```python
from build123d import *

# Parameters (mm, degrees)
F0_R     = 20
F1_DEPTH = 5
F2_W     = 5
F2_H     = 7.376282
F2_H_2   = 5
F3_DEPTH = 2


with BuildPart() as f1:
    # F0 (on Right) → F1 (new body)
    with BuildSketch(Plane.YZ):
        with BuildLine():
            Line((3.688141, 0), (3.688141, 32.210336))
            ThreePointArc((3.688141, 32.210336), (0, 75.898988), (-3.688141, 32.210336))
            Line((-3.688141, 32.210336), (-3.688141, 0))
            Line((-3.688141, 0), (3.688141, 0))
        make_face()
        with Locations((0, 53.898988)):
            Circle(F0_R, mode=Mode.SUBTRACT)
    extrude(amount=F1_DEPTH)

    # F2 (on Top) → F3 (join)
    with BuildSketch(Plane.XY):
        with Locations((2.5, 0)):
            Rectangle(F2_W, F2_H)
        with Locations((2.5, -6.188141)):
            Rectangle(F2_W, F2_H_2)
        with Locations((2.5, 6.188141)):
            Rectangle(F2_W, F2_H_2)
    extrude(amount=F3_DEPTH)


solid = f1.part
```
The model under review builds one solid part; all positions refer to its coordinate system, in mm. A direction names the side the tool comes from. Round coordinates to 2 decimals unless told otherwise and drop trailing zeros. Order: outer loops, then holes, each group sorted by start corner. A loop starts at its lowest first (then second) coordinate and runs counter-clockwise, first axis right, second up.
(1) Take a section at B-B, the plane z = 44. State the section outline as (x, y) points.
Working result:
outline: (0, -19.65) - (5, -19.65) - (5, -17.38) - (0, -17.38) - close; (0, 17.38) - (5, 17.38) - (5, 19.65) - (0, 19.65) - close
(2) For P1, Ø1.6, axis at x = 2, z = 1, coming from the +Y side; P2, Ø3, axis at x = 4, z = 61, coming from the +Y side; P3, Ø1, axis at x = 1.5, y = -2, coming from the -Z side; P4, Ø0.6, axis at x = 3, z = 0.5, coming from the -Y side, all flat-tipped, find the tip position at first contact; note any pin that passes through.
Working result:
P1: stops at y = 8.69
P2: stops at y = 21.28
P3: stops at z = 0
P4: stops at y = -8.69
(3) Take a section at A-A, the plane y = 0. State the section outline as (x, z) points.
Working result:
outline: (0, 0) - (5, 0) - (5, 33.9) - (0, 33.9) - close; (0, 73.9) - (5, 73.9) - (5, 75.9) - (0, 75.9) - close
(4) Mouldability with a two-part tool opening along Z and no side actions: class faces 6 (the face through (5, 0, 32)), 7 (the face through (2, 0, 0)), 8 (the face through (2, 6, 2)) as released by +Z, released by -Z, zero draft, split by the parting line, or undercut.
Working result:
face 6: zero draft
face 7: released by -Z
face 8: undercut
(5) Take a section at C-C, the plane x = 1.45. State the section outline as (y, z) points, plus the area to 3 significant figures.
Working result:
outline: (-8.69, 0) - (8.69, 0) - (8.69, 2) - (3.69, 2) - (3.69, 32.21) arc R22 ccw (long way) to (-3.69, 32.21) - (-3.69, 2) - (-8.69, 2) - close; hole circle Ø40 at (0, 53.9)
area: 520 mm2
(6) Take a section at D-D, the plane z = 11.5. State the section outline as (x, y) points.
Working result:
outline: (0, -3.69) - (5, -3.69) - (5, 3.69) - (0, 3.69) - close
(7) Wall thickness on L1, parallel to Z at x = 2.55, y = 0; L2, parallel to Z at x = 1.2, y = -7; L3, parallel to Y at x = 3.15, z = 21.5: over which ranges is each line inside the solid? List them lowest first.
Working result:
L1: z = 0 to 33.9, 73.9 to 75.9
L2: z = 0 to 2, 33.04 to 35.16, 72.63 to 74.76
L3: y = -3.69 to 3.69
(8) Tool access review of faces 1 (the face through (2, 8.688, 1)), 2 (the face through (2, -3.688, 17)), 3 (the face through (2, -8.688, 1)), 4 (the face through (2, 3.688, 17)), 5 (the face through (0, 0, 32)): name each direction out of +Z, -Z, +X, -X, +Y, -Y from which nothing blocks a thin tool from reaching the whole face with its end or side.
Working result:
face 1: -Z, +X, -X, +Y
face 2: +X, -X, -Y
face 3: -Z, +X, -X, -Y
face 4: +X, -X, +Y
face 5: +Z, -Z, -X, +Y, -Y
